Here's the drawing with two shaded views (mm, measured from the low corner). I have some questions. A direction names the side the tool comes from. Coordinates: 2 decimals unless noted, no trailing zeros. Write each loop counter-clockwise with the first axis right and the second up, starting at its lowest first coordinate (ties: lowest second). Pieces come first, ordered by that corner, then holes. Notation, with made-up numbers: (79, 47) -> (105, 47) arc R17 cw to (105, 67) -> close; hole circle Ø3 at (40.5, 82.25). An arc over 180 degrees is marked (long way). Put each result on its own line as item: value. Start each with the question number.
Item 1: I need wall thicknesses on line 1 (X direction, y = 5.75, z = 25); line 2 (X direction, y = 25, z = 15); line 3 (Z direction, x = 55, y = 2). Which ranges of each line are inside material? Lowest first, please. Write a range as [from, to].
Item 2: I want a section at B-B, the plane z = 25. List the corners of the cut face in (x, y) for me.
Item 3: If we mould it in two halves opening along X, with no side actions, what happens to the marked faces 4, 5 and 6? For each: released by +X, released by -X, zero draft, split by the parting line, or undercut.
Item 4: I want a section at A-A, the plane y = 8.5. List the corners of the cut face in (x, z) for me.
Item 5: I want a section at C-C, the plane x = 55. List the corners of the cut face in (y, z) for me (1 decimal).
Item 6: For pin 1 (16 mm diameter, centred on y = 25.5, z = 20.5, fed in from +X); pin 2 (10 mm diameter, centred on x = 53, z = 11, fed in from +Y); pin 3 (1 mm diameter, centred on x = 62, z = 16.5, fed in from +Y), each with a flat end and sliding along its axis, tell me the tip position at first contact or that it passes through.
Item 7: I want a section at D-D, the plane x = 38.5. List the corners of the cut face in (y, z) for me, then the cut area to 3 significant figures.
Item 8: On a 3-axis mill with a long thin cutter (end or side, diameter ignored), from which of +Z, -Z, +X, -X, +Y, -Y can I reach the whole of each face in a straight line? I mean the marked faces 1, 2 and 3. Say none if no direction works.
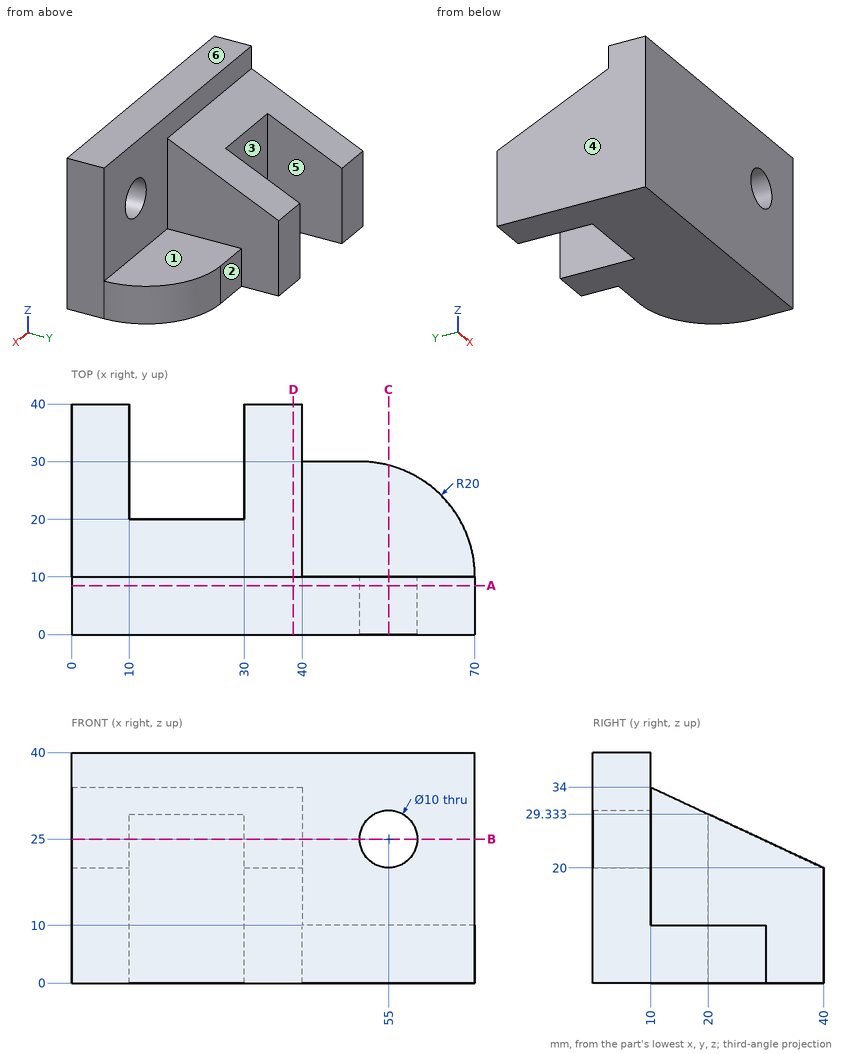
Calculated:
1. line 1: x = [0, 50], [60, 70]
1. line 2: x = [0, 10], [30, 40]
1. line 3: z = [0, 20], [30, 40]
2. outline: (0, 0) -> (50, 0) -> (50, 10) -> (40, 10) -> (40, 29.29) -> (30, 29.29) -> (30, 20) -> (10, 20) -> (10, 29.29) -> (0, 29.29) -> close; (60, 0) -> (70, 0) -> (70, 10) -> (60, 10) -> close
3. face 4: released by -X
3. face 5: undercut
3. face 6: zero draft
4. outline: (0, 0) -> (70, 0) -> (70, 40) -> (0, 40) -> close; hole circle Ø10 at (55, 25)
5. outline: (0, 0) -> (29.4, 0) -> (29.4, 10) -> (10, 10) -> (10, 20) -> (0, 20) -> close; (0, 30) -> (10, 30) -> (10, 40) -> (0, 40) -> close
6. pin 1: stops at x = 40
6. pin 2: stops at y = 30
6. pin 3: stops at y = 10
7. outline: (0, 0) -> (40, 0) -> (40, 20) -> (10, 34) -> (10, 40) -> (0, 40) -> close
7. area: 1,210 mm2
8. face 1: +Z, +X, +Y
8. face 2: +Z, -Z, +X, +Y
8. face 3: +Z, -Z, +Y
